from build123d import *

# Parameters (mm, degrees)
F0_R     = 34.2116613635
F1_DEPTH = 25.4
F2_R     = 57.5601591622
F3_DEPTH = 25.4
F5_D     = 6.35


with BuildPart() as f1:
    # F0 (on Right) → F1 (new body)
    with BuildSketch(Plane.YZ):
        Circle(F0_R)
    extrude(amount=F1_DEPTH)

    # F2 (on Front) → F3 (join)
    with BuildSketch(Plane.XZ):
        with Locations((26.8488749862, 0)):
            Circle(F2_R)
    extrude(amount=F3_DEPTH)

    # F5 (through all)
    with Locations(Plane(origin=(0, 0, 0), x_dir=(0, 1, 0), z_dir=(-1, 0, 0))):
        with Locations((22.584579885, 3.1673496123)):
            Hole(F5_D / 2)


solid = f1.part
Can you work these out from the model? Positions are in its coordinate system, mm. A direction names the side the tool comes from. Coordinates: 2 decimals unless noted, no trailing zeros. Write each loop counter-clockwise with the first axis right and the second up, starting at its lowest first coordinate (ties: lowest second). Pieces come first, ordered by that corner, then holes. Notation, with made-up numbers: M 19.25,40.5 L 70.25,40.5 A27 ccw 70.25,69.5 Z; hole C 73,82 d3. An arc over 180 degrees is marked long. Use one line per item in the form item = value.
Q1. I need wall thicknesses on line 1 along X through (y, z) = (-12, -0.5); line 2 along Y through (x, z) = (61.5, 5); line 3 along Z through (x, y) = (36, -23.5). Which ranges of each line are inside material? Lowest first, please. Write a range as from..to.
Model answer:
line_1 = -30.71..84.41
line_2 = -25.4..0
line_3 = -56.83..56.83
Q2. For P1, Ø4, axis at x = -2, y = -3, coming from the +Z side; P2, Ø9.5, axis at y = -30, z = -5, coming from the -X side; P3, Ø6, axis at y = 8, z = -22, coming from the +X side, each with a flat end and sliding along its axis, tell me the tip position at first contact or that it passes through.
Model answer:
P1 = 50.91
P2 = -30.58
P3 = 25.4
Q3. If we section it at A-A (x = 18.5): Write out the boundary of the cut face in (y, z) (3 decimals).
Model answer:
outline = M -25.4,-56.951 L 0,-56.951 L 0,-34.212 A34.212 ccw 0,34.212 L 0,56.951 L -25.4,56.951 L -25.4,22.919 A34.212 ccw -25.4,-22.919 Z; hole C 22.585,-3.167 d6.35
Q4. If we section it at D-D (x = 31): Write out the boundary of the cut face in (y, z).
Model answer:
outline = M -25.4,-57.41 L 0,-57.41 L 0,57.41 L -25.4,57.41 Z
Q5. If we section it at B-B (z = -29.5): Write out the boundary of the cut face in (x, y), then the cut area to 3 significant figures.
Model answer:
outline = M -22.58,-25.4 L 76.27,-25.4 L 76.27,0 L 25.4,0 L 25.4,17.33 L 0,17.33 L 0,0 L -22.58,0 Z
area = 2,950 mm^2
Q6. For faces 5 (the cylindrical face through (12.52, -34.21, 0.35)), 6 (the flat face through (25.4, -29, 0)), 7 (the flat face through (0, -29, 0)), 8 (the flat face through (25.4, 13, 0)), which set-ups out of +Z, -Z, +X, -X, +Y, -Y let a thin tool reach every point of the face, with its end or its side?
Model answer:
face_5 = +X, -X, -Y
face_6 = +Z, -Z, +X, -Y
face_7 = +Z, -Z, -X, -Y
face_8 = +Z, -Z, +X, +Y
Q7. We'd pull the mould along Y, two halves only. Please class faces 1 (the cylindrical face through (12.878, 25.757, -3.307)), 2 (the flat face through (0, 13, 0)), 3 (the flat face through (26, 0, 1)), 4 (the flat face through (26, -25.4, 1)): +Y half, -Y half, draft (parallel to the pull), parting line (faces both ways), or undercut.
Model answer:
face_1 = undercut
face_2 = draft
face_3 = +Y half
face_4 = -Y half
Q8. If we section it at C-C (y = 4): Write out the boundary of the cut face in (x, z).
Model answer:
outline = M 0,-33.98 L 25.4,-33.98 L 25.4,33.98 L 0,33.98 Z
